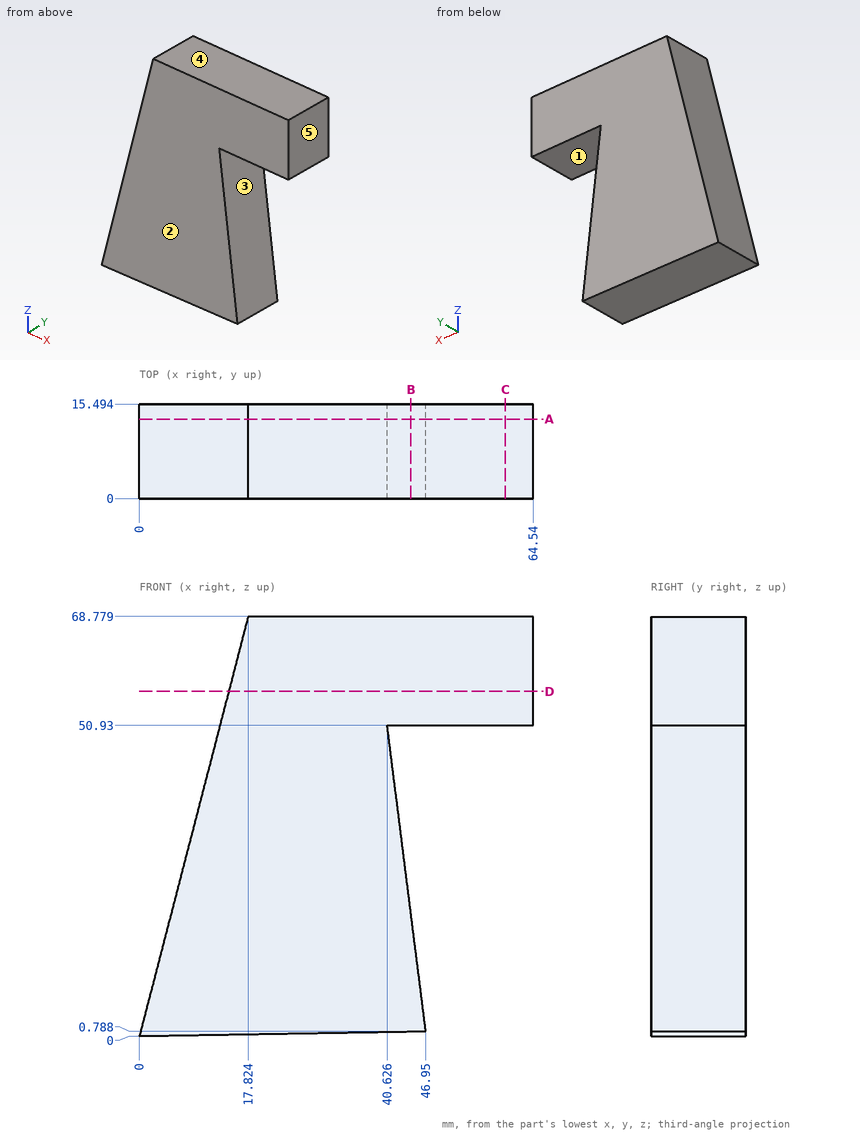
Study the drawing (mm; zero at the part's minimum x, y, z) and answer. A direction names the side the tool comes from. Give positions to 0.01 mm unless a question says otherwise; leave off trailing zeros. Write each loop counter-clockwise with the first axis right and the second up, starting at its lowest first coordinate (ties: lowest second). Pieces come first, ordered by that corner, then holes.
Item 1: Section A-A, the plane y = 13 is taken. Write down the section's boundary in (x, z).
Item 2: Determine the mould class of the marked faces 3, 4 and 5 for opening direction Z: released by +Z, released by -Z, zero draft, split by the parting line, or undercut.
Item 3: Find the intervals of material crossed by line 1 along Z through (x, y) = (61, 2.5); line 2 along X through (y, z) = (10.75, 14) (1 decimal); line 3 along X through (y, z) = (7.5, 20), in increasing order.
Item 4: Section B-B, the plane x = 44.5 is taken. Write down the section's boundary in (y, z), plus the area to 3 significant figures.
Item 5: Section C-C, the plane x = 60 is taken. Write down the section's boundary in (y, z), plus the area to 3 significant figures.
Item 6: Flat-ended cylindrical pins translate along their axes: P1, Ø2, axis at y = 7, z = 51.5, coming from the -X side; P2, Ø1, axis at y = 10.5, z = 55.5, coming from the -X side; P3, Ø8, axis at y = 9.5, z = 21.5, coming from the -X side (1 decimal). Find the tip coordinate at first contact, or state that the pin passes through.
Item 7: Which of the six approach directions +Z, -Z, +X, -X, +Y, -Y give full straight-line access (tool end or side, diameter ignored) to the marked faces 1 and 2?
Item 8: Section D-D, the plane z = 56.5 is taken. Write down the section's boundary in (x, y).
Completed:
1. outline: (0, 0) - (46.95, 0.79) - (40.63, 50.93) - (64.54, 50.93) - (64.54, 68.78) - (17.82, 68.78) - close
2. face 3: undercut
2. face 4: released by +Z
2. face 5: zero draft
3. line 1: z = 50.93 to 68.78
3. line 2: x = 3.6 to 45.3
3. line 3: x = 5.18 to 44.53
4. outline: (0, 0.75) - (15.49, 0.75) - (15.49, 20.22) - (0, 20.22) - close; (0, 50.93) - (15.49, 50.93) - (15.49, 68.78) - (0, 68.78) - close
4. area: 578 mm2
5. outline: (0, 50.93) - (15.49, 50.93) - (15.49, 68.78) - (0, 68.78) - close
5. area: 277 mm2
6. P1: stops at x = 13.09
6. P2: stops at x = 14.25
6. P3: stops at x = 4.5
7. face 1: +X, +Y, -Y
7. face 2: +Z, -Z, +X, -X, -Y
8. outline: (14.64, 0) - (64.54, 0) - (64.54, 15.49) - (14.64, 15.49) - close
